Geometry check sheet. Reference: the model listing, model coordinates, mm. Face numbers are marked on the shaded views. A direction names the side the tool comes from. Round coordinates to 2 decimals unless told otherwise and drop trailing zeros. Write each loop counter-clockwise with the first axis right and the second up, starting at its lowest first coordinate (ties: lowest second). Pieces come first, ordered by that corner, then holes. Notation, with made-up numbers: (66.25, -25) -> (105.25, -25) arc R24 ccw to (105.25, 11) -> close; hole circle Ø4 at (64, -19.5). An arc over 180 degrees is marked (long way). Put each result on its own line as item: value. Start each with the question number.
from build123d import *

# Parameters (mm, degrees)
F0_R     = 5.08
F1_DEPTH = 7.62
F2_R     = 8.032786
F3_DEPTH = 5.08
F4_R     = 2.636804
F5_R     = 0.508
F7_DEPTH = 4.1148


with BuildPart() as f1:
    # F0 (on Front) → F1 (new body)
    with BuildSketch(Plane.XZ):
        with BuildLine():
            ThreePointArc((0, -12.7), (8.980256, -8.980256), (12.7, 0))
            ThreePointArc((12.7, 0), (0, 12.7), (-12.7, 0))
            ThreePointArc((-12.7, 0), (-8.980256, -8.980256), (0, -12.7))
        make_face()
        Circle(F0_R, mode=Mode.SUBTRACT)
        with BuildLine():
            ThreePointArc((0, -12.7), (-8.980256, -8.980256), (-12.7, 0))
            ThreePointArc((-12.7, 0), (-13.8923, -2.978256), (-16.315987, -5.08))
            Line((-16.315987, -5.08), (-50.8, -5.08))
            Line((-50.8, -5.08), (-50.8, -12.7))
            Line((-50.8, -12.7), (0, -12.7))
        make_face()
    extrude(amount=F1_DEPTH)

    # F2 (on face) → F3 (cut)
    with BuildSketch(Plane.XZ.offset(7.62)):
        with BuildLine():
            Line((-25.4, -7.62), (-50.8, -7.62))
            Line((-50.8, -7.62), (-50.8, -10.16))
            Line((-50.8, -10.16), (-25.4, -10.16))
            Line((-25.4, -10.16), (-25.4, -11.176))
            Line((-25.4, -11.176), (-5.420324, -11.176))
            ThreePointArc((-5.420324, -11.176), (-4.39868, -10.322378), (-3.079561, -10.142513))
            ThreePointArc((-3.079561, -10.142513), (6.727909, 8.190818), (-9.351117, -4.991079))
            ThreePointArc((-9.351117, -4.991079), (-9.532285, -6.092003), (-10.523605, -6.604))
            Line((-10.523605, -6.604), (-10.551615, -6.604))
            Line((-10.551615, -6.604), (-25.4, -6.604))
            Line((-25.4, -6.604), (-25.4, -7.62))
        make_face()
        Circle(F2_R, mode=Mode.SUBTRACT)
    extrude(amount=-F3_DEPTH, mode=Mode.SUBTRACT)

    # F4
    f4_edges = [f1.edges().sort_by_distance(p)[0] for p in [
        (-50.8, -3.81, -5.08),
        (-50.8, -3.81, -12.7),
    ]]
    fillet(f4_edges, radius=F4_R)

    # F5
    f5_edges = [f1.edges().sort_by_distance(p)[0] for p in [
        (-5.08, 0, 0),
    ]]
    fillet(f5_edges, radius=F5_R)

    # F6 (on Front) → F7 (join)
    with BuildSketch(Plane.XZ):
        with BuildLine():
            ThreePointArc((-40.439792, -12.663556), (-38.240899, -15.451491), (-39.844185, -18.619642))
            ThreePointArc((-39.844185, -18.619642), (-40.724568, -19.661956), (-39.844185, -20.704271))
            ThreePointArc((-39.844185, -20.704271), (-35.908664, -20.084477), (-32.122858, -18.84345))
            ThreePointArc((-32.122858, -18.84345), (-27.401871, -14.325342), (-21.076703, -12.684218))
            Line((-21.076703, -12.684218), (-40.439792, -12.663556))
        make_face()
    extrude(amount=F7_DEPTH)


solid = f1.part
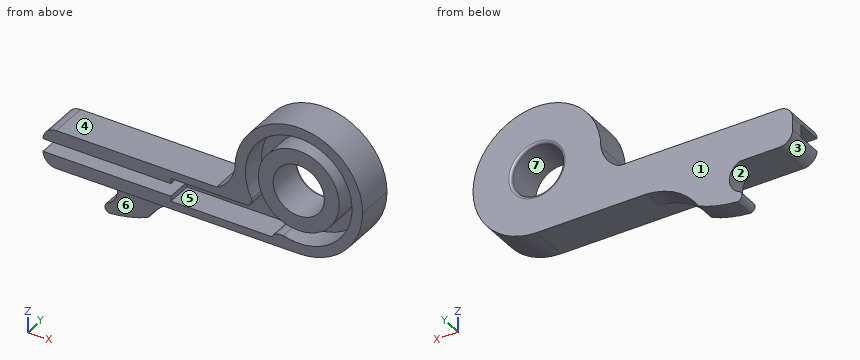
(1) Sectioned sample at C-C (y = -1.5). Record the cut outline in (x, z).
(2) Go/stop test with flat-tipped pins: pin 1 Ø3 at (x, y) = (-24, -1.5) entering from +Z; pin 2 Ø2 at (y, z) = (-2, 0) entering from -X; pin 3 Ø2.5 at (x, y) = (-17, -6.5) entering from -Z. Record where each tip stops, or that it passes through.
(3) Sectioned sample at A-A (y = -5). Record the cut outline in (x, z), and give its area (3 significant figures).
(4) Material ranges on L1, parallel to Z at x = 0, y = -3.5; L2, parallel to Z at x = -18, y = -3; L3, parallel to Z at x = -36.5, y = -4.5, recorded low to high. Write a range as from..to.
(5) Set-up check for the marked faces 4, 5, 6 and 7: record each of +Z, -Z, +X, -X, +Y, -Y from which the full face is reachable in a straight line by a thin tool's end or side.
(6) Sectioned sample at B-B (x = -17.5). Record the cut outline in (y, z), and give its area (3 significant figures).
(7) Mould release check, pull along Z, two halves, no side actions. Record for the marked faces 1, 2 and 3: +Z half, -Z half, draft (parallel to the pull), parting line (faces both ways), or undercut.
(8) Sectioned sample at D-D (x = -26). Record the cut outline in (y, z).
Found:
1. outline: (-50.8, -10.06) arc R2.64 ccw to (-48.16, -12.7) -> (-40.34, -12.7) arc R3.3 cw to (-39.84, -18.62) arc R1.06 ccw to (-39.84, -20.7) arc R24.84 ccw to (-32.12, -18.84) arc R12.96 cw to (-21.73, -12.7) -> (0, -12.7) arc R12.7 ccw (long way) to (-12.7, 0) arc R6.81 cw to (-16.32, -5.08) -> (-48.16, -5.08) arc R2.64 ccw to (-50.8, -7.72) -> close; hole circle Ø10.16 at (0, 0)
2. pin 1: z = -5.08
2. pin 2: x = -12.92
2. pin 3: z = -12.7
3. outline: (-50.8, -10.16) arc R2.64 ccw to (-48.16, -12.7) -> (0, -12.7) arc R12.7 ccw (long way) to (-12.7, 0) arc R6.81 cw to (-16.32, -5.08) -> (-48.16, -5.08) arc R2.64 ccw to (-50.8, -7.62) -> (-25.4, -7.62) -> (-25.4, -6.6) -> (-10.52, -6.6) arc R1.24 ccw to (-9.35, -4.99) arc R10.6 cw (long way) to (-3.08, -10.14) arc R2.41 ccw to (-5.42, -11.18) -> (-25.4, -11.18) -> (-25.4, -10.16) -> close; circle Ø16.07 at (0, 0); hole circle Ø10.16 at (0, 0)
3. area: 449 mm2
4. L1: -12.7..-10.6, -8.03..-5.08, 5.08..8.03, 10.6..12.7
4. L2: -12.7..-11.18, -6.6..-5.08
4. L3: -12.7..-10.16, -7.62..-5.08
5. face 4: +Z, -X, +Y, -Y
5. face 5: -Y
5. face 6: -Z, +X, -X, -Y
5. face 7: +Y, -Y
6. outline: (-7.62, -12.7) -> (0, -12.7) -> (0, -5.08) -> (-7.62, -5.08) -> (-7.62, -6.6) -> (-2.54, -6.6) -> (-2.54, -11.18) -> (-7.62, -11.18) -> close
6. area: 34.8 mm2
7. face 1: draft
7. face 2: undercut
7. face 3: -Z half
8. outline: (-7.62, -12.7) -> (-4.11, -12.7) -> (-4.11, -13.65) -> (0, -13.65) -> (0, -5.08) -> (-7.62, -5.08) -> (-7.62, -7.62) -> (-2.54, -7.62) -> (-2.54, -10.16) -> (-7.62, -10.16) -> close
